The listing builds one solid part. Answer for the finished solid, in the listing's coordinates (mm). A direction names the side the tool comes from. Coordinates: 2 decimals unless noted, no trailing zeros. Write each loop counter-clockwise with the first axis right and the second up, starting at its lowest first coordinate (ties: lowest second). Pieces come first, ordered by that corner, then holes.
from build123d import *
from build123d.topology import SkipClean

# Parameters (mm, degrees)
BOSS_EXTRUDE1_DEPTH = 22.5
SKETCH2_R           = 3
BOSS_EXTRUDE2_DEPTH = 2
SKETCH3_OUTSIDE_W   = 33.712
SKETCH3_OUTSIDE_H   = 24.512
SKETCH3_OUTSIDE_R   = 7.5
CUT_EXTRUDE1_DEPTH  = 20.7
SKETCH4_R           = 1.5
BOSS_EXTRUDE3_DEPTH = 7
SKETCH5_W           = 8.4
SKETCH5_H           = 5.786305447
BOSS_EXTRUDE4_DEPTH = 10


with BuildPart() as part:
    # Sketch1 → Boss-Extrude1 (new body)
    with BuildSketch(Plane.XY):
        with BuildLine():
            Line((-11.251411697, -1.686407058), (-3.416992222, -7.5))
            Line((-3.416992222, -7.5), (3.416992222, -7.5))
            Line((3.416992222, -7.5), (11.251411697, -1.686407058))
            ThreePointArc((11.251411697, -1.686407058), (11.993922619, 0.658993619), (10, 2.1))
            Line((10, 2.1), (7.2, 2.1))
            ThreePointArc((7.2, 2.1), (0, 7.5), (-7.2, 2.1))
            Line((-7.2, 2.1), (-10, 2.1))
            ThreePointArc((-10, 2.1), (-11.993922619, 0.658993619), (-11.251411697, -1.686407058))
        make_face()
    extrude(amount=BOSS_EXTRUDE1_DEPTH)

    # Sketch2 → Boss-Extrude2 (add)
    with BuildSketch(Plane.XY.offset(22.5)):
        Circle(SKETCH2_R)
    extrude(amount=BOSS_EXTRUDE2_DEPTH)

    # Sketch3 outside → Cut-Extrude1 (cut)
    with SkipClean():  # the faces are left unmerged after this step: merging them gives an invalid solid
        with BuildSketch(Plane(origin=(0, 0, 0), x_dir=(-1, 0, 0), z_dir=(0, 0, -1))):
            Rectangle(SKETCH3_OUTSIDE_W, SKETCH3_OUTSIDE_H)
            with Locations(Location((0, 0, 0), (0, 0, 16.260204708))):
                Circle(SKETCH3_OUTSIDE_R, mode=Mode.SUBTRACT)
        extrude(amount=-CUT_EXTRUDE1_DEPTH, mode=Mode.SUBTRACT)
    add(part.part.scale(1), mode=Mode.REPLACE)  # the faces are merged on a copy

    # Sketch4 → Boss-Extrude3 (add)
    with BuildSketch(Plane.XY.offset(24.5)):
        with Locations(Location((0, 0, 0), (0, 0, 180))):
            Circle(SKETCH4_R)
    extrude(amount=BOSS_EXTRUDE3_DEPTH)

    # Sketch5 → Boss-Extrude4 (add)
    with BuildSketch(Plane(origin=(0, 0, 0), x_dir=(-1, 0, 0), z_dir=(0, 0, -1))):
        with Locations((0, 9.106847276)):
            Rectangle(SKETCH5_W, SKETCH5_H)
    extrude(amount=-BOSS_EXTRUDE4_DEPTH)


solid = part.part
1. Section D-D on z = 25.5 is taken. Give the vertices of the cut face in (x, y).
Results found:
outline: circle Ø3 at (0, 0)
2. Section B-B on z = 15 is taken. Give the vertices of the cut face in (x, y).
Results found:
outline: circle Ø15 at (0, 0)
3. A tool of negligible diameter and unlimited length cuts with its end or side. For faces 1 (the cylindrical face through (-1.43, -0.45, 27.95)), 2 (the flat face through (9, 2.1, 22)), 3 (the flat face through (-4.2, 9, 5)), from which of +Z, -Z, +X, -X, +Y, -Y can it reach the whole face along a straight path? Write none if from no direction.
Results found:
face 1: +Z
face 2: +Z, -Z, +X, +Y
face 3: +Z, -Z, -X, +Y
4. Section A-A on y = 0 is taken. Give the vertices of the cut face in (x, z).
Results found:
outline: (-12.1, 20.7) - (-7.5, 20.7) - (-7.5, 0) - (7.5, 0) - (7.5, 20.7) - (12.1, 20.7) - (12.1, 22.5) - (3, 22.5) - (3, 24.5) - (1.5, 24.5) - (1.5, 31.5) - (-1.5, 31.5) - (-1.5, 24.5) - (-3, 24.5) - (-3, 22.5) - (-12.1, 22.5) - close
5. Section C-C on x = 2.5 is taken. Give the vertices of the cut face in (y, z).
Results found:
outline: (-7.5, 20.7) - (-7.07, 20.7) - (-7.07, 0) - (12, 0) - (12, 10) - (7.07, 10) - (7.07, 22.5) - (1.66, 22.5) - (1.66, 24.5) - (-1.66, 24.5) - (-1.66, 22.5) - (-7.5, 22.5) - close
6. Find the intervals of material crossed by L1, parallel to Z at x = 0, y = 6.25; L2, parallel to Z at x = 0, y = 11; L3, parallel to X at y = 11, z = 8, in increasing order.
Results found:
L1: z = 0 to 22.5
L2: z = 0 to 10
L3: x = -4.2 to 4.2
7. Flat-ended cylindrical pins translate along their axes: P1, Ø2, axis at x = -4.5, y = -5.5, coming from the +Z side; P2, Ø4, axis at x = -2, z = 16, coming from the +Y side; P3, Ø3, axis at y = 1, z = 25, coming from the -X side. Find the tip coordinate at first contact, or state that the pin passes through.
Results found:
P1: stops at z = 22.5
P2: stops at y = 7.5
P3: stops at x = -3
